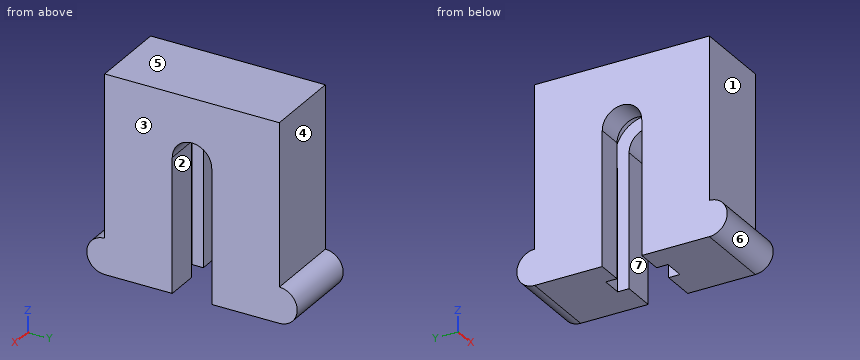
Autodesk Fusion 360 part; units mm, degrees
sketch "Boceto1" plane through (0, 0, 0) normal (0, 0, 1) x (1, 0, 0)
sketch "Boceto2" plane through (0, 0, 0) normal (1, 0, 0) x (0, 1, 0)
  line L0 (0, 0) -> (68.5, 0)
  line L1 (68.5, 0) -> (68.5, 77.5)
  line L2 (68.5, 77.5) -> (0, 77.5)
  line L3 (0, 77.5) -> (0, 0)
  line L4 (0, 0) -> (26.5, 0)
  line L5 (68.5, 0) -> (42, 0)
  line L6 (0, 0) -> (0, 7)
  line L7 (68.5, 0) -> (68.5, 7)
  circle A0 centre (0, 7) radius 7
  circle A1 centre (68.5, 7) radius 7
  line L8 (68.5, 14) -> (68.5, 52.5)
  line L9 (26.5, 0) -> (42, 0)
  line L10 (42, 0) -> (42, 52.5)
  line L11 (26.5, 52.5) -> (26.5, 0)
  circle A2 centre (34.25, 52.5) radius 7.75
  line L12 (26.5, 52.5) -> (26.5, 0)
  line L13 (42, 52.5) -> (42, 0)
  line L14 (26.5, 52.5) -> (42, 52.5)
  dimension "d2" = 77.5
  dimension "d3" = 26.5
  dimension "d4" = 26.5
  dimension "d9_1" = 15.5
  dimension "d89" = 68.5
sketch "Boceto3" plane through (0, 0, 0) normal (1, 0, 0) x (0, 1, 0)
extrude "Extruir2" add sketch "Boceto2" along normal blind 31 contours L0 L1 L2 L3 L4 L5 A0 A1 L8 L10 L11 A2 L12 L13 | L3 L6 A0 | L3 L6 A0 | L1 L7 A1 | L1 L7 A1
sketch "Boceto4" plane through (0, 26.5, 0) normal (0, 1, 0) x (-1, 0, 0)
  line L0 (0, 0) -> (0, 52.5)
  line L1 (0, 52.5) -> (-31, 52.5)
  line L2 (-31, 52.5) -> (-31, 0)
  line L3 (-31, 0) -> (0, 0)
  line L4 (-31, 0) -> (-21, 0)
  line L5 (-21, 0) -> (-13, 0)
  line L6 (-13, 0) -> (0, 0)
  dimension "d14_1" = 10
  dimension "d15_1" = 8
sketch "Boceto5" plane through (0, 0, 0) normal (0, 0, -1) x (1, 0, 0)
  line L0 (0, -42) -> (0, -68.5)
  line L1 (0, -68.5) -> (31, -68.5)
  line L2 (31, -68.5) -> (31, -42)
  line L3 (31, -42) -> (0, -42)
  line L4 (31, -42) -> (31, -26.5)
  line L5 (31, -26.5) -> (31, -34.25)
  line L6 (31, -34.25) -> (0, -34.25)
  line L7 (0, -34.25) -> (0, -22.05)
  line L8 (0, -34.25) -> (0, -46.45)
  line L9 (0, -34.25) -> (31, -34.25)
  line L10 (0, -34.25) -> (0, -22.05)
  line L11 (0, -22.05) -> (31, -22.05)
  line L12 (31, -22.05) -> (31, -34.25)
  line L13 (0, -46.45) -> (31, -46.45)
  line L14 (31, -46.45) -> (31, -22.05)
  line L15 (0, -22.05) -> (10, -22.05)
  line L16 (10, -22.05) -> (18.1, -22.05)
  line L17 (10, -22.05) -> (18.1, -22.05)
  line L18 (18.1, -22.05) -> (18.1, -46.45)
  line L19 (18.1, -46.45) -> (10, -46.45)
  line L20 (10, -46.45) -> (10, -22.05)
  dimension "d16_1" = 12.2
  dimension "d17_1" = 12.2
  dimension "d18_1" = 10
  dimension "d19" = 8.1
  dimension "d20" = 8.1
extrude "Extruir3" cut sketch "Boceto5" against normal blind 52.5 contours L3 L6 L9 L18 L20 | L3 L13 L18 L19 L20 | L6 L9 L11 L16 L17 L18 L20
ref_plane "PlanoDeObra1" through (10, 44.225, 26.25) normal (1, 0, 0) x (0, 1, 0)
sketch "Boceto6" plane through (10, 44.975, 26.25) normal (1, 0, 0) x (0, 1, 0)
  circle A0 centre (-9.975, 26.25) radius 12.55
  dimension "d24_1" = 25.1
extrude "Extruir4" cut sketch "Boceto6" along normal blind 8.1
sketch "Boceto7" plane through (0, 0, 0) normal (0, 0, -1) x (1, 0, 0)
  line L0 (18.1, -22.05) -> (18.1, -26.5)
  line L1 (18.1, -26.5) -> (31, -26.5)
  line L2 (31, -26.5) -> (31, 0)
  line L3 (31, 0) -> (0, 0)
  line L4 (0, 0) -> (0, -26.5)
  line L5 (0, -26.5) -> (10, -26.5)
  line L6 (10, -26.5) -> (10, -22.05)
  line L7 (10, -22.05) -> (18.1, -22.05)
Model file for the job. Use its own axes, mm. Face numbers are marked on the shaded views. A direction names the side the tool comes from. Coordinates: 2 decimals unless noted, no trailing zeros. Order: outer loops, then holes, each group sorted by start corner. A loop starts at its lowest first (then second) coordinate and runs counter-clockwise, first axis right, second up. Notation, with made-up numbers: (-8, -11.5) -> (5, -11.5) arc R33 cw to (5, 26.5) -> close; hole circle Ø3 at (66, 17.25). An arc over 180 degrees is marked (long way). Return JSON: item names as keys, results as strings.
Item 1: Slice it at B-B (x = 25). Write the cut outline in (y, z).
Model answer:
{"outline": "(0, 0) -> (26.5, 0) -> (26.5, 52.5) arc R7.75 cw to (42, 52.5) -> (42, 0) -> (68.5, 0) arc R7 ccw to (68.5, 14) -> (68.5, 77.5) -> (0, 77.5) -> (0, 14) arc R7 ccw to start"}
Item 2: Wall check: line 1 along Y through (x, z) = (15, 52); line 2 along Y through (x, z) = (3, 24); line 3 along Z through (x, y) = (13, 35). Give the ranges that are in metal, low to high. Write a range as from..to.
Model answer:
{"line 1": "y = 0..22.05, 47.54..68.5", "line 2": "y = 0..26.5, 42..68.5", "line 3": "z = 65.05..77.5"}
Item 3: 3-axis set-ups, long thin cutter, end or side, ignore diameter. For the marked faces 1, 2, 3 and 4: which of +Z, -Z, +X, -X, +Y, -Y reach the whole face in a straight line?
Model answer:
{"face 1": "+Z, +X, -X, -Y", "face 2": "-Z, +X, -X", "face 3": "+Z, -Z, +X, +Y, -Y", "face 4": "+Z, +X, -X, +Y"}
Item 4: Mould opens along Y. For the marked faces 5, 6 and 7 say: pulls with the +Y half, pulls with the -Y half, needs draft (parallel to the pull), parting line crosses it, or undercut.
Model answer:
{"face 5": "needs draft", "face 6": "pulls with the -Y half", "face 7": "undercut"}
Item 5: Slice it at C-C (y = 35). Write the cut outline in (x, z).
Model answer:
{"outline": "(0, 60.21) -> (10, 60.21) -> (10, 65.05) -> (18.1, 65.05) -> (18.1, 60.21) -> (31, 60.21) -> (31, 77.5) -> (0, 77.5) -> close"}
Item 6: Pin check, flat tips, straight feed: P1, Ø1, axis at x = 26, z = 40.5, coming from the +Y side; P2, Ø3, axis at x = 7, z = 16.5, coming from the -Y side. Stop position of each tip, or through.
Model answer:
{"P1": "stops at y = 68.5", "P2": "stops at y = 0"}
Item 7: Slice it at A-A (z = 7). Write the cut outline in (x, y).
Model answer:
{"outline": "(0, -7) -> (31, -7) -> (31, 26.5) -> (18.1, 26.5) -> (18.1, 22.05) -> (10, 22.05) -> (10, 26.5) -> (0, 26.5) -> close; (0, 42) -> (10, 42) -> (10, 46.45) -> (18.1, 46.45) -> (18.1, 42) -> (31, 42) -> (31, 75.5) -> (0, 75.5) -> close"}
Item 8: Slice it at D-D (z = 25.5). Write the cut outline in (x, y).
Model answer:
{"outline": "(0, 0) -> (31, 0) -> (31, 26.5) -> (18.1, 26.5) -> (18.1, 22.05) -> (10, 22.05) -> (10, 26.5) -> (0, 26.5) -> close; (0, 42) -> (10, 42) -> (10, 46.45) -> (18.1, 46.45) -> (18.1, 42) -> (31, 42) -> (31, 68.5) -> (0, 68.5) -> close"}
